Read the model definition and answer for the solid it produces. Units are mm, in the model's axes. A direction names the side the tool comes from. Coordinates: 2 decimals unless noted, no trailing zeros. Loops run counter-clockwise (first coordinate to the right, second up) from the corner with the lowest first, then second, coordinate; pieces in that order, holes last. Notation, with made-up numbers: (54, 27.5) - (59, 27.5) arc R15 ccw to (59, 33.5) - close; hole circle Ø9 at (31.25, 18). An arc over 180 degrees is marked (long way). One line per question, with ' | ' between items. Start each with the question number.
```python
from build123d import *

# Parameters (mm, degrees)
PAD_DEPTH       = 10
SKETCH001_R     = 1.5
SKETCH001_W     = 2
SKETCH001_H     = 1
POCKET_DEPTH    = 10.001
SKETCH002_R     = 1.4
PAD001_DEPTH    = 10
FILLET_R        = 1
FILLET001_R     = 1
FILLET002_R     = 1
FILLET003_R     = 3
SKETCH003_R     = 1.9
POCKET001_DEPTH = 6
FILLET004_R     = 0.5
FILLET005_R     = 1
SKETCH004_R     = 3.2
POCKET002_DEPTH = 3
SKETCH005_R     = 1.3
POCKET003_DEPTH = 15.001


with BuildPart() as part:
    # Sketch → Pad (new body)
    with BuildSketch(Plane.XY):
        Polygon((0, 4), (-5, 4), (-5, 1), (2, 1), (2, -1), (-5, -1), (-5, -4), (0, -4), (0, -10), (10, -10), (10, 10), (0, 10), align=None)
    extrude(amount=PAD_DEPTH)

    # Sketch001 (on Face14 of Pad) → Pocket (cut, through all)
    with BuildSketch(Plane.XY.offset(10)):
        with Locations((2, 0)):
            Circle(SKETCH001_R)
        with Locations((1, 4.5)):
            Rectangle(SKETCH001_W, SKETCH001_H)
    extrude(amount=-POCKET_DEPTH, mode=Mode.SUBTRACT)

    # Sketch002 (on Face4 of Pocket) → Pad001 (join)
    with BuildSketch(Plane.XY.offset(10)):
        with Locations((-3, 3)):
            Circle(SKETCH002_R)
        with Locations((-3, -3)):
            Circle(SKETCH002_R)
    extrude(amount=-PAD001_DEPTH)

    # Fillet
    fillet_edges = [part.edges().sort_by_distance(p)[0] for p in [
        (-5, 4, 5),
        (-5, 1, 5),
        (-5, -1, 5),
        (-5, -4, 5),
    ]]
    fillet(fillet_edges, radius=FILLET_R)

    # Fillet001
    fillet001_edges = [part.edges().sort_by_distance(p)[0] for p in [
        (0.881966, 1, 5),
        (0.881966, -1, 5),
    ]]
    fillet(fillet001_edges, radius=FILLET001_R)

    # Fillet002
    fillet002_edges = [part.edges().sort_by_distance(p)[0] for p in [
        (0, 5, 5),
        (0, -10, 5),
    ]]
    fillet(fillet002_edges, radius=FILLET002_R)

    # Fillet003
    fillet003_edges = [part.edges().sort_by_distance(p)[0] for p in [
        (10, -10, 5),
    ]]
    fillet(fillet003_edges, radius=FILLET003_R)

    # Sketch003 (on Face7 of Fillet003) → Pocket001 (cut)
    with BuildSketch(Plane(origin=(0, 10, 0), x_dir=(-1, 0, 0), z_dir=(0, 1, 0))):
        with Locations((-5, 5)):
            Circle(SKETCH003_R)
    extrude(amount=-POCKET001_DEPTH, mode=Mode.SUBTRACT)

    # Fillet004
    fillet004_edges = [part.edges().sort_by_distance(p)[0] for p in [
        (2, 4, 5),
    ]]
    fillet(fillet004_edges, radius=FILLET004_R)

    # Fillet005
    fillet005_edges = [part.edges().sort_by_distance(p)[0] for p in [
        (0, 10, 5),
        (10, 10, 5),
    ]]
    fillet(fillet005_edges, radius=FILLET005_R)

    # Sketch004 (on Face9 of Fillet005) → Pocket002 (cut)
    with BuildSketch(Plane.YZ.offset(10)):
        with Locations((0, 5)):
            Circle(SKETCH004_R)
    extrude(amount=-POCKET002_DEPTH, mode=Mode.SUBTRACT)

    # Sketch005 (on Face9 of Pocket002) → Pocket003 (cut, through all)
    with BuildSketch(Plane.YZ.offset(10)):
        with Locations((0, 5)):
            Circle(SKETCH005_R)
    extrude(amount=-POCKET003_DEPTH, mode=Mode.SUBTRACT)


solid = part.part
```
1) Find the intervals of material crossed by line 1 along Z through (x, y) = (5, 7.7); line 2 along Z through (x, y) = (7.8, 0); line 3 along Y through (x, z) = (-4, 9.5), in increasing order. Write a range as from..to.
2) The mould has two halves that part along Y. Classify faces 4 (the cylindrical face through (-4.83, -1.44, 5.07)), 5 (the flat face through (4, 0, 0)), 6 (the cylindrical face through (4.904, 0.6, 3.847)), 7 (the cylindrical face through (-3, 4.4, 5.1)): released by +Y, released by -Y, zero draft, split by the parting line, or undercut.
3) Which of the six approach directions +Z, -Z, +X, -X, +Y, -Y give full straight-line access (tool end or side, diameter ignored) to faces 1 (the flat face through (0, 4, 5)), 2 (the flat face through (-2, -1, 2)), 3 (the flat face through (5, 4, 5))?
4) The part is cut by section D-D on y = 8.75. Write down the section's boundary in (x, z).
5) The part is cut by section B-B on y = 0. Write down the section's boundary in (x, z), and give its area (3 significant figures).
6) The part is cut by section A-A on x = 5. Write down the section's boundary in (y, z), and give its area (3 significant figures).
7) Given pin 1 Ø3 at (x, z) = (4.5, 5) entering from +Y; pin 2 Ø2.5 at (x, z) = (5, 5) entering from +Y; pin 3 Ø3.5 at (y, z) = (0, 5) entering from -X; pin 4 Ø4 at (y, z) = (-7, 7) entering from -X, each flat-ended and moving along its own axis, determine where each tip first touches the part or whether it passes through.
Answer below:
1) line 1: 0..3.1, 6.9..10 | line 2: 0..1.8, 8.2..10 | line 3: -4..-1, 1..4
2) face 4: undercut | face 5: zero draft | face 6: undercut | face 7: released by +Y
3) face 1: +Z, -Z | face 2: +Z, -Z, -X | face 3: +Y
4) outline: (0, 0) - (10, 0) - (10, 10) - (0, 10) - close; hole circle Ø3.8 at (5, 5)
5) outline: (3.5, 0) - (10, 0) - (10, 1.8) - (7, 1.8) - (7, 3.7) - (3.5, 3.7) - close; (3.5, 6.3) - (7, 6.3) - (7, 8.2) - (10, 8.2) - (10, 10) - (3.5, 10) - close | area: 36.7 mm2
6) outline: (-10, 0) - (10, 0) - (10, 3.1) - (4, 3.1) - (4, 6.9) - (10, 6.9) - (10, 10) - (-10, 10) - close; hole circle Ø2.6 at (0, 5) | area: 172 mm2
7) pin 1: y = 10 | pin 2: y = 4 | pin 3: x = -4.97 | pin 4: x = 0
